Autodesk Inventor part; units mm, degrees
ref_plane "YZ Plane" through (0, 0, 0) normal (1, 0, 0) x (0, 1, 0)
ref_plane "XZ Plane" through (0, 0, 0) normal (0, 1, 0) x (-1, 0, 0)
ref_plane "XY Plane" through (0, 0, 0) normal (0, 0, 1) x (1, 0, 0)
sketch "sketch1--base" plane through (0, 0, 0) normal (0, 1, 0) x (-1, 0, 0)
  line L0 (-18.2322, -18.2322) -> (18.2322, 18.2322) construction
  line L1 (21.7082, -21.7082) -> (-21.7082, 21.7082) construction
  line L2 (-20, -20) -> (20, -20) construction
  line L3 (20, -20) -> (20, 20) construction
  line L4 (20, 20) -> (-20, 20) construction
  line L5 (-20, 20) -> (-20, -20) construction
  line L6 (-20, -20) -> (20, 20) construction
  line L7 (20, -20) -> (-20, 20) construction
  line L8 (-21.7678, -21.7678) -> (21.7678, 21.7678) construction
  line L9 (21.7678, -21.7678) -> (-21.7678, 21.7678) construction
  circle A0 centre (-20, 20) radius 2.5 construction
  circle A1 centre (20, 20) radius 2.5 construction
  circle A2 centre (20, -20) radius 2.5 construction
  circle A3 centre (-20, -20) radius 2.5 construction
  arc A4 (17.5, 20) -> (20, 17.5) centre (20, 20) ccw
  arc A5 (20, -17.5) -> (17.5, -20) centre (20, -20) ccw
  arc A6 (-20, 17.5) -> (-17.5, 20) centre (-20, 20) ccw
  arc A7 (-17.5, -20) -> (-20, -17.5) centre (-20, -20) ccw
  line L10 (-17.5, -20) -> (17.5, -20)
  line L11 (-20, -17.5) -> (-20, 17.5)
  line L12 (0, -20) -> (0, 20) construction
  line L13 (20, 0) -> (-20, 0) construction
  line L14 (20, -17.5) -> (20, 17.5)
  line L15 (17.5, 20) -> (-17.5, 20)
  point P0 (0, 0)
  point P1 (20, 0)
  dimension "d6" = 40
  dimension "screw__diameter" = 5
  dimension "d24" = 40
sketch "sketch2--component" plane through (0, 0, 0) normal (0, 1, 0) x (-1, 0, 0)
  circle A0 centre (0, 0) radius 18.5
  circle A1 centre (0, 0) radius 15.8 construction
  circle A2 centre (0, -15.8) radius 1.5
  circle A3 centre (0, 0) radius 17.3 construction
  circle A4 centre (13.6832, -7.9) radius 1.5
  circle A5 centre (13.6832, 7.9) radius 1.5
  circle A6 centre (0, 15.8) radius 1.5
  circle A7 centre (-13.6832, 7.9) radius 1.5
  circle A8 centre (-13.6832, -7.9) radius 1.5
  circle A9 centre (0, 0) radius 6
  dimension "d40" = 37
  dimension "d41" = 1.2
  dimension "d42" = 3
  dimension "d45" = 360
  dimension "d49" = 12
sketch "Sketch3--union" plane through (0, 0, 0) normal (0, 1, 0) x (-1, 0, 0)
  circle A0 centre (13.6832, 7.9) radius 1.5
  circle A1 centre (13.6832, -7.9) radius 1.5
  circle A2 centre (0, -15.8) radius 1.5
  circle A3 centre (-13.6832, -7.9) radius 1.5
  circle A4 centre (-13.6832, 7.9) radius 1.5
  circle A5 centre (0, 15.8) radius 1.5
  circle A6 centre (0, 0) radius 20 construction
  line L0 (20, -20) -> (20, 20) construction
  arc A7 (0, -20) -> (0, 20) centre (0, 0) ccw
  line L1 (0, -20) -> (0, 20) construction
  line L2 (0, 20) -> (-150, 20)
  line L3 (-150, -20) -> (0, -20)
  line L4 (-20, 20) -> (-20, -20) construction
  line L5 (-20, 20) -> (-150, 0) construction
  line L6 (-20, 0) -> (-150, 20) construction
  line L7 (20, 0) -> (-20, 0) construction
  circle A8 centre (20, 20) radius 2.5 construction
  circle A9 centre (0, 0) radius 6
  line L8 (-132.5, 10) -> (-37.5, 10) construction
  line L9 (-132.5, 10) -> (-37.5, 10) construction
  line L10 (-150, 7.5) -> (-40, 7.5)
  line L11 (-40, 12.5) -> (-150, 12.5)
  arc A10 (-40, 7.5) -> (-40, 12.5) centre (-40, 10) ccw
  line L12 (-150, 20) -> (-150, 12.5)
  line L13 (-150, 7.5) -> (-150, 0)
  line L14 (-150, -7.5) -> (-40, -7.5)
  line L15 (-40, -12.5) -> (-150, -12.5)
  arc A11 (-40, -12.5) -> (-40, -7.5) centre (-40, -10) ccw
  line L16 (-150, -20) -> (-150, -12.5)
  line L17 (-150, -7.5) -> (-150, 0)
  point P0 (-85, 10)
  point P1 (-85, 10)
  point P2 (-85, 10)
  dimension "d52" = 2.5
  dimension "d53" = 130
  dimension "d54" = 20
extrude "Extrusion3--base" add sketch "Sketch3--union" along normal blind 6
equation "\"d6\" = module__size"
equation "\"d24\" = d6"
equation "\"d50\" = module__height"
equation "\"module__height\" = 6"
equation "\"module__size\" = 40"
properties part number "work-area--holder--motor"
For this review, take the finished solid that the model builds, in its own axes (mm). A direction names the side the tool comes from. Round coordinates to 2 decimals unless told otherwise and drop trailing zeros. Loops run counter-clockwise (first coordinate to the right, second up) from the corner with the lowest first, then second, coordinate; pieces in that order, holes last. Notation, with made-up numbers: (82, -30) - (127, -30) arc R4 ccw to (127, -25) - close; hole circle Ø10 at (60.25, -18.75). An arc over 180 degrees is marked (long way). One line per item, written item: value. Start each with the question number.
Item 1: For faces 4 (the flat face through (66, 0, 0)), 5 (the flat face through (94, 3, 12.5)), list the 3-axis set-ups (+Z, -Z, +X, -X, +Y, -Y) from which the entire face can be reached by the end or side of a thin tool; tool diameter is ignored.
Item 2: Take a section at C-C (z = -4.5). Give the boundary of the cut face in (x, y), plus the area to 3 significant figures.
Item 3: Take a section at B-B (y = 1.05). Give the boundary of the cut face in (x, z).
Item 4: The part is to be moulded in two halves that separate along Z. For faces 1 (the flat face through (76, 3, -20)), 2 (the flat face through (96, 3, -7.5)), 3 (the flat face through (74, 3, 20)), say which applies: +Z half, -Z half, draft (parallel to the pull), parting line (faces both ways), or undercut.
Item 5: Clearance check with a flat-ended pin moving along its axis: pin 1 Ø5 at (x, z) = (13.68, 7.9) entering from -Y. State where the tip first meets the part, or that it passes through.
Item 6: For L1, parallel to Z at x = 95, y = 3.15; L2, parallel to Z at x = 0, y = 2.25; L3, parallel to X at y = 1.35, z = -13, list the stretches that pass through material, from the lowest coordinate up.
Item 7: Take a section at A-A (x = 83.5). Give the boundary of the cut face in (y, z).
Answer below:
1. face 4: +Z, -Z, +X, -X, -Y
1. face 5: +X, +Y, -Y
2. outline: (-19.49, 0) - (-3.97, 0) - (-3.97, 6) - (-19.49, 6) - close; (3.97, 0) - (150, 0) - (150, 6) - (3.97, 6) - close
2. area: 969 mm2
3. outline: (0, -20) - (150, -20) - (150, -12.5) - (40, -12.5) arc R2.5 cw to (40, -7.5) - (150, -7.5) - (150, 7.5) - (40, 7.5) arc R2.5 cw to (40, 12.5) - (150, 12.5) - (150, 20) - (0, 20) arc R20 ccw to start; hole circle Ø3 at (-13.68, -7.9); hole circle Ø3 at (-13.68, 7.9); hole circle Ø12 at (0, 0); hole circle Ø3 at (0, -15.8); hole circle Ø3 at (0, 15.8); hole circle Ø3 at (13.68, -7.9); hole circle Ø3 at (13.68, 7.9)
4. face 1: -Z half
4. face 2: undercut
4. face 3: +Z half
5. pin 1: stops at y = 0
6. L1: z = -20 to -12.5, -7.5 to 7.5, 12.5 to 20
6. L2: z = -20 to -17.3, -14.3 to -6, 6 to 14.3, 17.3 to 20
6. L3: x = -15.2 to 150
7. outline: (0, -20) - (6, -20) - (6, -12.5) - (0, -12.5) - close; (0, -7.5) - (6, -7.5) - (6, 7.5) - (0, 7.5) - close; (0, 12.5) - (6, 12.5) - (6, 20) - (0, 20) - close
